Source: CAD feature listing. Evaluate the final solid. Frame: model axes, mm. A direction names the side the tool comes from. Give positions to 0.01 mm unless a question says otherwise; leave off trailing zeros. Loops run counter-clockwise (first coordinate to the right, second up) from the corner with the lowest first, then second, coordinate; pieces in that order, holes last. Notation, with made-up numbers: (66, 75) -> (73, 75) arc R8 cw to (73, 89) -> close; hole circle Ø8 at (36, 25.5). An arc over 180 degrees is marked (long way). Return JSON: item names as keys, results as strings. Group by question number.
```python
from build123d import *

# Parameters (mm, degrees)
SKETCH1_R           = 10
BOSS_EXTRUDE1_DEPTH = 3
SKETCH2_R           = 5.6
BOSS_EXTRUDE2_DEPTH = 28
CUT_EXTRUDE1_DEPTH  = 7
CUT_EXTRUDE2_REACH  = 14.5
SKETCH4_R           = 1.5
FILLET1_R           = 3
FILLET1_2_R         = 1.5


with BuildPart() as part:
    # Sketch1 → Boss-Extrude1 (new body)
    with BuildSketch(Plane.XY):
        Circle(SKETCH1_R)
    extrude(amount=BOSS_EXTRUDE1_DEPTH)

    # Sketch2 → Boss-Extrude2 (add)
    with BuildSketch(Plane(origin=(0, 0, 0), x_dir=(-1, 0, 0), z_dir=(0, 0, -1))):
        Circle(SKETCH2_R)
    extrude(amount=BOSS_EXTRUDE2_DEPTH)

    # Sketch3 → Cut-Extrude1 (cut)
    with BuildSketch(Plane(origin=(0, 0, -28), x_dir=(-1, 0, 0), z_dir=(0, 0, -1))):
        with BuildLine():
            Line((2.5, 0), (2.5, 6.663171691))
            ThreePointArc((2.5, 6.663171691), (8.066213365, -0.537352556), (2.5, -7.737876802))
            Line((2.5, -7.737876802), (2.5, 0))
        make_face()
        with BuildLine():
            Line((-2.5, 0), (-2.5, 6.663171691))
            ThreePointArc((-2.5, 6.663171691), (-7.668145551, -0.537352556), (-2.5, -7.737876802))
            Line((-2.5, -7.737876802), (-2.5, 0))
        make_face()
    extrude(amount=-CUT_EXTRUDE1_DEPTH, mode=Mode.SUBTRACT)

    # Sketch4 → Cut-Extrude2 (cut, up to next)
    with BuildSketch(Plane(origin=(2.5, 0, 0), x_dir=(0, 0, -1), z_dir=(1, 0, 0)), mode=Mode.PRIVATE) as cut_extrude2_sk1:
        with Locations((24.5, 0)):
            Circle(SKETCH4_R)
    cut_extrude2_tool1 = extrude(cut_extrude2_sk1.sketch, amount=-CUT_EXTRUDE2_REACH, mode=Mode.PRIVATE) & part.part
    add(cut_extrude2_tool1.solids().sort_by_distance((2.5, 0, -24.5))[0], mode=Mode.SUBTRACT)

    # Fillet1
    fillet1_edges = [part.edges().sort_by_distance(p)[0] for p in [
        (5.6, 0, 0),
    ]]
    fillet(fillet1_edges, radius=FILLET1_R)

    # Fillet1 2
    fillet1_2_edges = [part.edges().sort_by_distance(p)[0] for p in [
        (2.5, 0, -21),
        (-2.5, 0, -21),
        (2.5, 0, -28),
        (-2.5, 0, -28),
    ]]
    fillet(fillet1_2_edges, radius=FILLET1_2_R)


solid = part.part
```
1) Reachability of faces 4 (the face through (-2.5, -1, -23)), 5 (the face through (5.595, 0.246, -12.547)), 6 (the face through (2.5, -1, -23)) from +Z, -Z, +X, -X, +Y, -Y: full face, straight path, thin tool, end or side. Return the list, or none.
2) Cut plane A-A on z = -24.5. Return loops of the section in (x, y), then the cut area to 3 significant figures.
3) Mould query, pull axis Y, two halves, no side actions, for faces 1 (the face through (-2.17, -9.76, 1.48)), 2 (the face through (0, 0, -23)), 3 (the face through (2.93, 0.07, -21.45)). Classes: released by +Y, released by -Y, zero draft, split by the parting line, or undercut.
4) Cut plane D-D on z = -19. Return loops of the section in (x, y).
5) Cut plane B-B on x = 0. Return loops of the section in (y, z), then the cut area to 3 significant figures.
6) Material intervals for line 1 (Z direction, x = 4, y = -8.25); line 2 (Y direction, x = -0.8, z = -24.5); line 3 (X direction, y = -3, z = -24), sorted ascending.
7) Contact query for flat-ended pins moving along their axis: P1, Ø1, axis at x = 3.5, z = -5.5, coming from the +Y side; P2, Ø0.8, axis at x = 4.5, y = 1, coming from the -Z side; P3, Ø12, axis at x = -7, z = -5.5, coming from the -Y side. Output: stop coordinate, or through.
8) Cut plane C-C on y = 0. Return loops of the section in (x, z).
Calculated:
{
 "1": {"face 4": "-Z, -X, +Y, -Y", "face 5": "-Z", "face 6": "-Z, +X, +Y, -Y"},
 "2": {"outline": "(-2.5, -5.01) arc R5.6 ccw to (2.5, -5.01) -> (2.5, -1.5) -> (-2.5, -1.5) -> close; (-2.5, 1.5) -> (2.5, 1.5) -> (2.5, 5.01) arc R5.6 ccw to (-2.5, 5.01) -> close", "area": "39.1 mm2"},
 "3": {"face 1": "split by the parting line", "face 2": "undercut", "face 3": "zero draft"},
 "4": {"outline": "circle Ø11.2 at (0, 0)"},
 "5": {"outline": "(-10, 0) -> (-8.6, 0) arc R3 cw to (-5.6, -3) -> (-5.6, -28) -> (5.6, -28) -> (5.6, -3) arc R3 cw to (8.6, 0) -> (10, 0) -> (10, 3) -> (-10, 3) -> close; hole circle Ø3 at (0, -24.5)", "area": "370 mm2"},
 "6": {"line 1": "0 to 3", "line 2": "-5.54 to -1.5, 1.5 to 5.54", "line 3": "-2.5 to 2.5"},
 "7": {"P1": "y = 4.73", "P2": "z = -21", "P3": "y = -8.88"},
 "8": {"outline": "(-10, 0) -> (-8.6, 0) arc R3 cw to (-5.6, -3) -> (-5.6, -21) -> (-4, -21) arc R1.5 cw to (-2.5, -22.5) -> (-2.5, -23) -> (2.5, -23) -> (2.5, -22.5) arc R1.5 cw to (4, -21) -> (5.6, -21) -> (5.6, -3) arc R3 cw to (8.6, 0) -> (10, 0) -> (10, 3) -> (-10, 3) -> close; (-2.5, -26.5) arc R1.5 ccw to (-1, -28) -> (1, -28) arc R1.5 ccw to (2.5, -26.5) -> (2.5, -26) -> (-2.5, -26) -> close"}
}
